Geometry: final body of the model. Coordinates: model frame, mm. Give positions to 0.01 mm unless a question says otherwise; leave off trailing zeros. Order: outer loops, then holes, each group sorted by start corner. A loop starts at its lowest first (then second) coordinate and runs counter-clockwise, first axis right, second up. Notation, with made-up numbers: (-10, 85) -> (47, 85) arc R15 ccw to (47, 93) -> close; hole circle Ø8 at (-11, 86). An arc over 180 degrees is marked (long way). Answer in a Markdown table with one row per item. Add a question column.
Q1. Line query: line 1 along Z through (x, y) = (0, 4.5); line 2 along X through (y, z) = (6, 1.5). Output: solid intervals per line, ascending. Write a range as from..to.
Q2. Cut plane B-B on z = 0. Return the cut outline in (x, y) (1 decimal), and give its area (3 significant figures).
Q3. Cut plane A-A on x = 0. Return the cut outline in (y, z) (1 decimal).
Q4. Contact query for flat-ended pins moving along their axis: P1, Ø3, axis at y = 2.5, z = -3.5, coming from the +X side; P2, Ø3, axis at x = -1.5, y = 5.5, coming from the +Z side; P3, Ø5, axis at x = 2.5, y = 3, coming from the -Z side. Output: stop coordinate, or through.
Q5. Cut plane C-C on y = 1. Return the cut outline in (x, z) (1 decimal).
Q6. Cut plane D-D on z = -2.5. Return the cut outline in (x, y) (3 decimals), and give its area (3 significant figures).
Q7. Pull-direction query (Z, two-part tool) for faces 1 (the face through (1, 1.905, -4)), 2 (the face through (0.632, 4.829, -1.525)), 3 (the face through (-0.83, 5.77, 3.72)); classes: +Z half, -Z half, draft (parallel to the pull), parting line (faces both ways), or undercut.
Autodesk Inventor part; units mm, degrees
ref_plane "YZ Plane" through (0, 0, 0) normal (1, 0, 0) x (0, 1, 0)
ref_plane "XZ Plane" through (0, 0, 0) normal (0, 1, 0) x (-1, 0, 0)
ref_plane "XY Plane" through (0, 0, 0) normal (0, 0, 1) x (1, 0, 0)
sketch "Sketch1" plane through (0, 0, 0) normal (0, 1, 0) x (-1, 0, 0)
  circle A0 centre (0, 0) radius 4.7625
  dimension "d0" = 9.525
extrude "Extrusion1" add sketch "Sketch1" along normal blind 9.525
sketch "Sketch2" plane through (0, 9.525, 0) normal (0, 1, 0) x (1, 0, 0)
  circle A0 centre (0, 0) radius 6.35
  circle A1 centre (0, 0) radius 3.81
  dimension "d3" = 12.7
  dimension "d4" = 7.62
extrude "Extrusion2" cut sketch "Sketch2" against normal blind 7.62
sketch "Sketch3" plane through (0, 0, 0) normal (0, -1, 0) x (1, 0, 0)
  circle A0 centre (0, 0) radius 1.5777
hole "Hole1" at (0, 0, 0) direction (0, 1, 0) diameter 3.302 end through all
properties part number "feet type 2 part 1" material "Brass, Soft Yellow"
Completed:
| question | item | result |
|---|---|---|
| 1 | line 1 | z = -3.81..-1.65, 1.65..3.81 |
| 1 | line 2 | x = -3.5..-0.69, 0.69..3.5 |
| 2 | outline | (-4.8, 0) -> (-1.7, 0) -> (-1.7, 9.5) -> (-3.8, 9.5) -> (-3.8, 1.9) -> (-4.8, 1.9) -> close; (1.7, 0) -> (4.8, 0) -> (4.8, 1.9) -> (3.8, 1.9) -> (3.8, 9.5) -> (1.7, 9.5) -> close |
| 2 | area | 44.8 mm² |
| 3 | outline | (0, -4.8) -> (1.9, -4.8) -> (1.9, -3.8) -> (9.5, -3.8) -> (9.5, -1.7) -> (0, -1.7) -> close; (0, 1.7) -> (9.5, 1.7) -> (9.5, 3.8) -> (1.9, 3.8) -> (1.9, 4.8) -> (0, 4.8) -> close |
| 4 | P1 | stops at x = 4.26 |
| 4 | P2 | stops at z = 3.81 |
| 4 | P3 | stops at z = -4.76 |
| 5 | outline | circle Ø9.5 at (0, 0); hole circle Ø3.3 at (0, 0) |
| 6 | outline | (-4.054, 0) -> (4.054, 0) -> (4.054, 1.905) -> (2.875, 1.905) -> (2.875, 9.525) -> (-2.875, 9.525) -> (-2.875, 1.905) -> (-4.054, 1.905) -> close |
| 6 | area | 59.3 mm² |
| 7 | face 1 | draft |
| 7 | face 2 | undercut |
| 7 | face 3 | parting line |
